Autodesk Inventor part; units mm, degrees
ref_plane "YZ Plane" through (0, 0, 0) normal (1, 0, 0) x (0, 1, 0)
ref_plane "XZ Plane" through (0, 0, 0) normal (0, 1, 0) x (-1, 0, 0)
ref_plane "XY Plane" through (0, 0, 0) normal (0, 0, 1) x (1, 0, 0)
sketch "スケッチ2" plane through (0, 0, 0) normal (0, 0, 1) x (1, 0, 0)
  line L0 (0, 0) -> (2.5, 0)
  line L1 (2.5, 0) -> (2.5, 150)
  line L2 (2.5, 150) -> (0, 150)
  line L3 (0, 150) -> (0, 0)
  line L4 (1.1, 0) -> (1.1, 6)
  line L5 (1.1, 6) -> (0, 6)
  line L6 (1.1, 150) -> (1.1, 154)
  line L7 (1.1, 154) -> (0, 154)
  line L8 (0, 154) -> (0, 150)
  dimension "d4" = 2.5
  dimension "d5" = 150
  dimension "d6" = 1.1
  dimension "d7" = 6
  dimension "d8" = 1.1
  dimension "d9" = 4
revolve "回転1" add sketch "スケッチ2" angle 360 about axis through (0, 150, 0) along (0, -1, 0) contours L4 L5 L3 L2 L1 L0 | L8 L7 L6 L2
properties part number "BaseSpacer_M3"
Could you check a few things on this model? Use its own coordinates, in mm. Give positions to 0.01 mm unless a question says otherwise; leave off trailing zeros. Loops run counter-clockwise (first coordinate to the right, second up) from the corner with the lowest first, then second, coordinate; pieces in that order, holes last. Notation, with made-up numbers: (-27, -15) -> (-21, -15) arc R24 cw to (-21, 24) -> close; hole circle Ø6 at (-13.5, -5.75). An arc over 180 degrees is marked (long way). Return JSON: item names as keys, results as strings.
Item 1: We'd pull the mould along Y, two halves only. Please class faces 1 (the cylindrical face through (-0.54, 76.05, 2.44)), 2 (the flat face through (1, 0, -1)), 3 (the flat face through (1, 150, -1)): +Y half, -Y half, draft (parallel to the pull), parting line (faces both ways), or undercut.
Geometry results:
{"face 1": "draft", "face 2": "-Y half", "face 3": "+Y half"}
Item 2: If we section it at A-A on x = 0: List the corners of the cut face in (y, z) for me, plus the area to 3 significant figures.
Geometry results:
{"outline": "(0, -2.5) -> (150, -2.5) -> (150, -1.1) -> (154, -1.1) -> (154, 1.1) -> (150, 1.1) -> (150, 2.5) -> (0, 2.5) -> (0, 1.1) -> (6, 1.1) -> (6, -1.1) -> (0, -1.1) -> close", "area": "746 mm²"}
Item 3: If we section it at C-C on y = 98: List the corners of the cut face in (x, z) for me.
Geometry results:
{"outline": "circle Ø5 at (0, 0)"}
Item 4: I need wall thicknesses on L1, parallel to Z at x = 0, y = 2.7; L2, parallel to Z at x = -0.1, y = 12.5; L3, parallel to Y at x = 0.55, z = -0.3. Which ranges of each line are inside material? Lowest first, please. Write a range as from..to.
Geometry results:
{"L1": "z = -2.5..-1.1, 1.1..2.5", "L2": "z = -2.5..2.5", "L3": "y = 6..154"}
Item 5: I'm going to push flat-ended pins straight in: pin 1 (2 mm diameter, centred on y = 74, z = -2, fed in from +X); pin 2 (3 mm diameter, centred on x = 2, y = 65.5, fed in from +Z); pin 3 (3 mm diameter, centred on x = 0.5, y = 65.5, fed in from -Z); pin 4 (1.1 mm diameter, centred on x = 0.5, z = 0, fed in from -Y). Where does each tip first touch, or does it pass through?
Geometry results:
{"pin 1": "stops at x = 2.29", "pin 2": "stops at z = 2.45", "pin 3": "stops at z = -2.5", "pin 4": "stops at y = 6"}
Item 6: If we section it at B-B on z = 0: List the corners of the cut face in (x, y) for me.
Geometry results:
{"outline": "(-2.5, 0) -> (-1.1, 0) -> (-1.1, 6) -> (1.1, 6) -> (1.1, 0) -> (2.5, 0) -> (2.5, 150) -> (1.1, 150) -> (1.1, 154) -> (-1.1, 154) -> (-1.1, 150) -> (-2.5, 150) -> close"}
